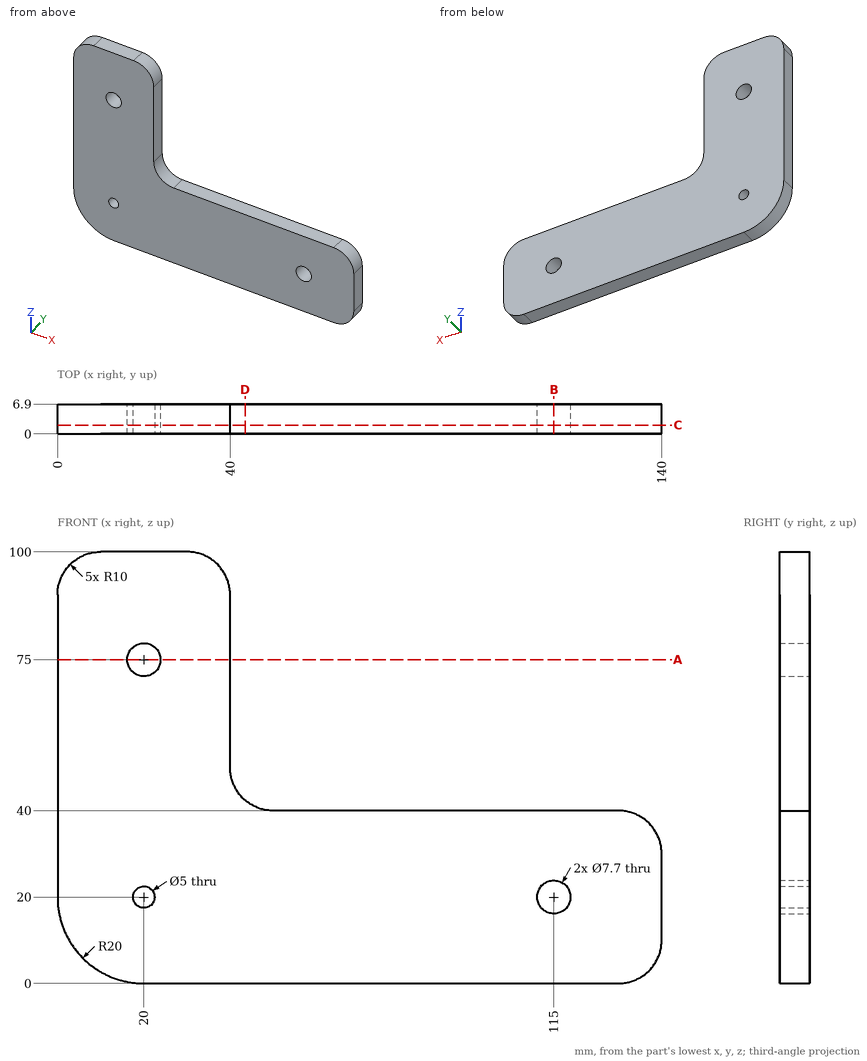
Can you work these out from the drawing? Everything is in mm from the part's minimum corner. Coordinates: 2 decimals unless noted, no trailing zeros. Loops run counter-clockwise (first coordinate to the right, second up) from the corner with the lowest first, then second, coordinate; pieces in that order, holes last. Notation, with made-up numbers: (61, -0.5) - (99, -0.5) arc R12 cw to (99, 7.5) - close; hole circle Ø11 at (41.5, 79.5). An arc over 180 degrees is marked (long way). Answer as CSV lines item,"result".
Q1. If we section it at D-D, the plane x = 43.5: Write out the boundary of the cut face in (y, z), and give its area (3 significant figures).
Response:
outline,"(0, 0) - (6.9, 0) - (6.9, 42.4) - (0, 42.4) - close"
area,"293 mm2"
Q2. If I drill on L1, parallel to Z at x = 20, y = 4.25; L2, parallel to X at y = 3.5, z = 20; L3, parallel to Z at x = 115, y = 2.75, over which ranges is the centre line in solid material (lowest first)? Write a range as [from, to].
Response:
L1,"[0, 17.5], [22.5, 71.15], [78.85, 100]"
L2,"[0, 17.5], [22.5, 111.15], [118.85, 140]"
L3,"[0, 16.15], [23.85, 40]"
Q3. For pin 1 (4.5 mm diameter, centred on x = 20, z = 75, fed in from -Y); pin 2 (2 mm diameter, centred on x = 70.5, y = 3.5, fed in from +Z); pin 3 (3.5 mm diameter, centred on y = 4.5, z = 73.5, fed in from +X), each with a flat end and sliding along its axis, tell me the tip position at first contact or that it passes through.
Response:
pin 1,"through"
pin 2,"z = 40"
pin 3,"x = 40"
Q4. If we section it at C-C, the plane y = 2: Write out the boundary of the cut face in (x, z).
Response:
outline,"(0, 20) arc R20 ccw to (20, 0) - (130, 0) arc R10 ccw to (140, 10) - (140, 30) arc R10 ccw to (130, 40) - (50, 40) arc R10 cw to (40, 50) - (40, 90) arc R10 ccw to (30, 100) - (10, 100) arc R10 ccw to (0, 90) - close; hole circle Ø7.7 at (20, 75); hole circle Ø5 at (20, 20); hole circle Ø7.7 at (115, 20)"
Q5. If we section it at B-B, the plane x = 115: Write out the boundary of the cut face in (y, z).
Response:
outline,"(0, 0) - (6.9, 0) - (6.9, 16.15) - (0, 16.15) - close; (0, 23.85) - (6.9, 23.85) - (6.9, 40) - (0, 40) - close"
Q6. If we section it at A-A, the plane z = 75: Write out the boundary of the cut face in (x, y).
Response:
outline,"(0, 0) - (16.15, 0) - (16.15, 6.9) - (0, 6.9) - close; (23.85, 0) - (40, 0) - (40, 6.9) - (23.85, 6.9) - close"
